Check sheet for the modelled part. Datum: model origin and axes. Units: mm. Face numbers are marked on the shaded views. A direction names the side the tool comes from. Round coordinates to 2 decimals unless told otherwise and drop trailing zeros. Order: outer loops, then holes, each group sorted by start corner. A loop starts at its lowest first (then second) coordinate and runs counter-clockwise, first axis right, second up.
```python
from build123d import *

# Parameters (mm, degrees)
BOSS_EXTRUDE1_DEPTH = 14
SKETCH1_3_R         = 2.5
BOSS_EXTRUDE2_DEPTH = 10
SKETCH3_R           = 2.5
CUT_EXTRUDE1_DEPTH  = 6


with BuildPart() as part:
    # Sketch1 → Boss-Extrude1 (new body)
    with BuildSketch(Plane(origin=(0, 0, 0), x_dir=(1, 0, 0), z_dir=(0, 1, 0))):
        Polygon((0, 4.618802154), (-4, 2.309401077), (-4, -2.309401077), (0, -4.618802154), (4, -2.309401077), (4, 2.309401077), align=None)
    extrude(amount=BOSS_EXTRUDE1_DEPTH)

    # Sketch1_3 → Boss-Extrude2 (add)
    with BuildSketch(Plane(origin=(0, 0, 0), x_dir=(1, 0, 0), z_dir=(0, 1, 0))):
        with Locations(Location((0, 0, 0), (0, 0, 270))):
            Circle(SKETCH1_3_R)
    extrude(amount=-BOSS_EXTRUDE2_DEPTH)

    # Sketch3 → Cut-Extrude1 (cut)
    with BuildSketch(Plane(origin=(0, 14, 0), x_dir=(1, 0, 0), z_dir=(0, 1, 0))):
        with Locations(Location((0, 0, 0), (0, 0, 270))):
            Circle(SKETCH3_R)
    extrude(amount=-CUT_EXTRUDE1_DEPTH, mode=Mode.SUBTRACT)


solid = part.part
```
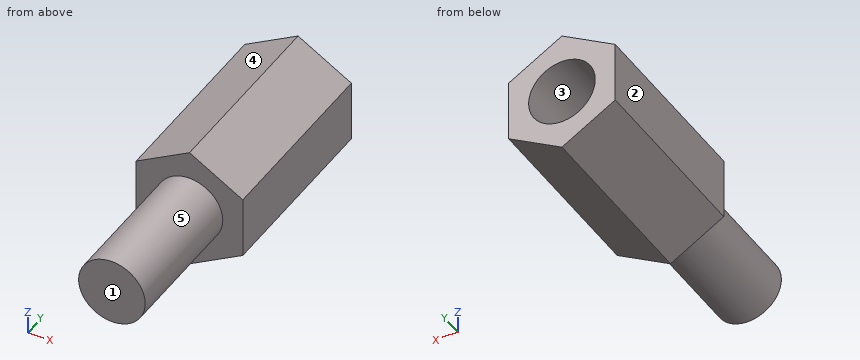
Item 1: Sectioned sample at C-C (y = 7). Record the cut outline in (x, z), and give its area (3 significant figures).
Answer:
outline: (-4, -2.31) - (0, -4.62) - (4, -2.31) - (4, 2.31) - (0, 4.62) - (-4, 2.31) - close
area: 55.4 mm2
Item 2: Scan lines: line 1 along X through (y, z) = (10.1, 0); line 2 along Y through (x, z) = (0.5, 3.75); line 3 along X through (y, z) = (10.25, -1.25). Record each from-to range of solid material in increasing order.
Answer:
line 1: x = -4 to -2.5, 2.5 to 4
line 2: y = 0 to 14
line 3: x = -4 to -2.17, 2.17 to 4
Item 3: Sectioned sample at B-B (x = -0.75). Record the cut outline in (y, z), and give its area (3 significant figures).
Answer:
outline: (-10, -2.38) - (0, -2.38) - (0, -4.19) - (14, -4.19) - (14, -2.38) - (8, -2.38) - (8, 2.38) - (14, 2.38) - (14, 4.19) - (0, 4.19) - (0, 2.38) - (-10, 2.38) - close
area: 136 mm2
Item 4: Access from +Z, -Z, +X, -X, +Y, -Y to the whole of each face (thin tool, end or side, straight path). Record for the marked faces 4 and 5.
Answer:
face 4: +Z, -X, +Y, -Y
face 5: -Y
Item 5: Sectioned sample at A-A (z = -1.5). Record the cut outline in (x, y).
Answer:
outline: (-4, 0) - (-2, 0) - (-2, -10) - (2, -10) - (2, 0) - (4, 0) - (4, 14) - (2, 14) - (2, 8) - (-2, 8) - (-2, 14) - (-4, 14) - close
Item 6: Go/stop test with flat-tipped pins: P1, Ø1.5, axis at x = 0, z = -1, coming from the +Y side; P2, Ø4, axis at y = 6.5, z = 3, coming from the +X side. Record where each tip stops, or that it passes through.
Answer:
P1: stops at y = 8
P2: stops at x = 4
Item 7: Sectioned sample at D-D (y = -6.75). Record the cut outline in (x, z).
Answer:
outline: circle Ø5 at (0, 0)
Item 8: Release check for a two-part mould opening along X. For the marked faces 1, 2 and 3 record: released by +X, released by -X, zero draft, split by the parting line, or undercut.
Answer:
face 1: zero draft
face 2: released by -X
face 3: undercut
